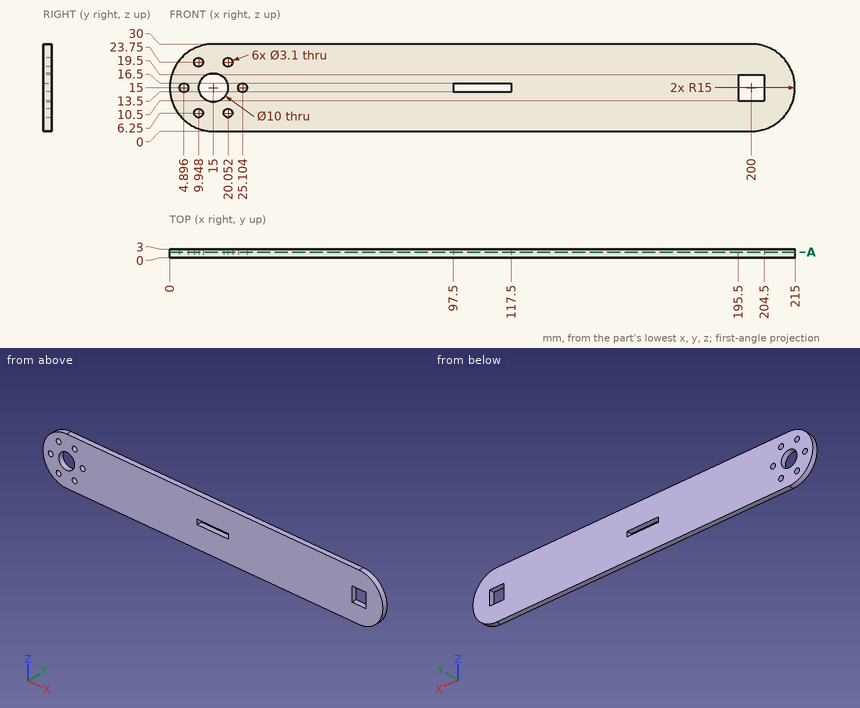
Source: three-view drawing plus pictorial views. Frame: mm from the lowest corner of the part. Round coordinates to 2 decimals unless told otherwise and drop trailing zeros. Use one line per item in the form item = value.
(1) Section A-A on y = 2. Count the separate pieces of the cut face and the enclosed holes in it, and give its area (3 significant figures).
Results list:
separate_pieces = 1
enclosed_holes = 9
area = 5,990 mm^2
(2) Ray query, probe 1 along X at (y, z) = (2.35, 17) (1 decimal); probe 2 along X at (y, z) = (0.45, 7) (1 decimal); probe 3 along Z at (x, y) = (110, 0.6). Return the intervals inside material, ascending. Write a range as [from, to].
Results list:
probe_1 = [0.1, 10.4], [19.6, 195.5], [204.5, 214.9]
probe_2 = [2.3, 8.6], [11.3, 18.7], [21.4, 212.7]
probe_3 = [0, 13.5], [16.5, 30]
(3) First-contact query: pin 1 Ø1.5 at (y, z) = (2, 8.5) entering from -X (1 decimal); pin 2 Ø1.9 at (x, z) = (25.1, 15) entering from -Y; pin 3 Ø0.9 at (y, z) = (1, 14) entering from +X. Flat tips, straight axial feed; report the tip coordinate or a pass-through.
Results list:
pin_1 = 1.1
pin_2 = through
pin_3 = 214.99
